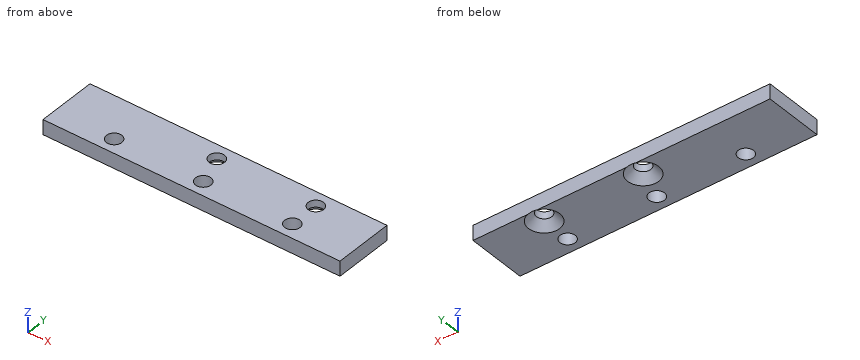
```python
from build123d import *

# Parameters (mm, degrees)
SKETCH_1_W      = 60
SKETCH_1_H      = 12
SKETCH_1_R      = 1.55
EXTRUDE_1_DEPTH = 3
CHAMFER_1_SIZE  = 1.6


with BuildPart() as part:
    # 草图1 → 凸台-拉伸1 (new body)
    with BuildSketch(Plane.XY):
        Rectangle(SKETCH_1_W, SKETCH_1_H)
        with Locations((18, 3)):
            Circle(SKETCH_1_R, mode=Mode.SUBTRACT)
        with Locations((-2, 3)):
            Circle(SKETCH_1_R, mode=Mode.SUBTRACT)
        with Locations((0, -3)):
            Circle(SKETCH_1_R, mode=Mode.SUBTRACT)
        with Locations((18, -3)):
            Circle(SKETCH_1_R, mode=Mode.SUBTRACT)
        with Locations((-18, -3)):
            Circle(SKETCH_1_R, mode=Mode.SUBTRACT)
    extrude(amount=EXTRUDE_1_DEPTH)

    # 倒角1
    # the kernel refuses this chamfer: 1.6 mm, written as the material it takes off along each edge
    with BuildSketch(Plane(origin=(18, 3, 0), x_dir=(1, 0, 0), z_dir=(0, -1, 0))) as chamfer_1_piece_1:
        Polygon((1.55, CHAMFER_1_SIZE), (1.55 + CHAMFER_1_SIZE, 0), (1.55, 0), align=None)
    revolve(axis=Axis((18, 3, 0), (0, 0, 1)), mode=Mode.SUBTRACT)
    with BuildSketch(Plane(origin=(-2, 3, 0), x_dir=(1, 0, 0), z_dir=(0, -1, 0))) as chamfer_1_piece_2:
        Polygon((1.55, CHAMFER_1_SIZE), (1.55 + CHAMFER_1_SIZE, 0), (1.55, 0), align=None)
    revolve(axis=Axis((-2, 3, 0), (0, 0, 1)), mode=Mode.SUBTRACT)


solid = part.part
```
Geometry: final body of the model. Coordinates: model frame, mm. Give positions to 0.01 mm unless a question says otherwise; leave off trailing zeros. Loops run counter-clockwise (first coordinate to the right, second up) from the corner with the lowest first, then second, coordinate; pieces in that order, holes last. Notation, with made-up numbers: (-14.5, -33) - (-8.5, -33) arc R24 ccw to (-8.5, -14) - close; hole circle Ø7 at (24, 1.25). An arc over 180 degrees is marked (long way). Answer as CSV lines item,"result". Start each with the question number.
(1) Section query B-B (z = 2.15). Output: boundary loops of the cut face in (x, y), and give its area (3 significant figures).
(2) Section query D-D (x = 18). Output: boundary loops of the cut face in (y, z), and give its area (3 significant figures).
(3) Section query A-A (y = 3). Output: boundary loops of the cut face in (x, z).
(4) Ray query, line 1 along Y through (x, z) = (18, 2.05); line 2 along Y through (x, z) = (17, 1.5); line 3 along X through (y, z) = (2.75, 1.95). Return the intervals inside material, ascending. Write a range as [from, to].
(5) Pin query (flat end, axial travel): P1, Ø1.9, axis at x = -18, y = -3, coming from the -Z side. Return the tip coordinate at first contact, or that it passes through.
(6) Section query C-C (x = -18). Output: boundary loops of the cut face in (y, z), and give its area (3 significant figures).
Worked answers:
1,outline,"(-30, -6) - (30, -6) - (30, 6) - (-30, 6) - close; hole circle Ø3.1 at (-18, -3); hole circle Ø3.1 at (-2, 3); hole circle Ø3.1 at (0, -3); hole circle Ø3.1 at (18, -3); hole circle Ø3.1 at (18, 3)"
1,area,"682 mm^2"
2,outline,"(-6, 0) - (-4.55, 0) - (-4.55, 3) - (-6, 3) - close; (-1.45, 0) - (-0.15, 0) - (1.45, 1.6) - (1.45, 3) - (-1.45, 3) - close; (4.55, 1.6) - (6, 0.15) - (6, 3) - (4.55, 3) - close"
2,area,"14.9 mm^2"
3,outline,"(-30, 0) - (-5.15, 0) - (-3.55, 1.6) - (-3.55, 3) - (-30, 3) - close; (-0.45, 1.6) - (1.15, 0) - (14.85, 0) - (16.45, 1.6) - (16.45, 3) - (-0.45, 3) - close; (19.55, 1.6) - (21.15, 0) - (30, 0) - (30, 3) - (19.55, 3) - close"
4,line 1,"y = [-6, -4.55], [-1.45, 1.45], [4.55, 6]"
4,line 2,"y = [-6, -4.18], [-1.82, 1.69], [4.31, 6]"
4,line 3,"x = [-30, -3.53], [-0.47, 16.47], [19.53, 30]"
5,P1,"passes through"
6,outline,"(-6, 0) - (-4.55, 0) - (-4.55, 3) - (-6, 3) - close; (-1.45, 0) - (6, 0) - (6, 3) - (-1.45, 3) - close"
6,area,"26.7 mm^2"
